The drawing under review shows one solid part. Ordinate dimensions are in mm from its lowest x, y, z. A direction names the side the tool comes from. Give positions to 0.01 mm unless a question says otherwise; leave off trailing zeros. Write each loop counter-clockwise with the first axis right and the second up, starting at its lowest first coordinate (ties: lowest second). Pieces come first, ordered by that corner, then holes. Notation, with made-up numbers: M -12.5,28.5 L 7.5,28.5 A9 ccw 7.5,45.5 Z; hole C -36,-12.75 d9. An arc over 180 degrees is marked long. Answer as a JSON object with one key per item and string values. Group by question number.
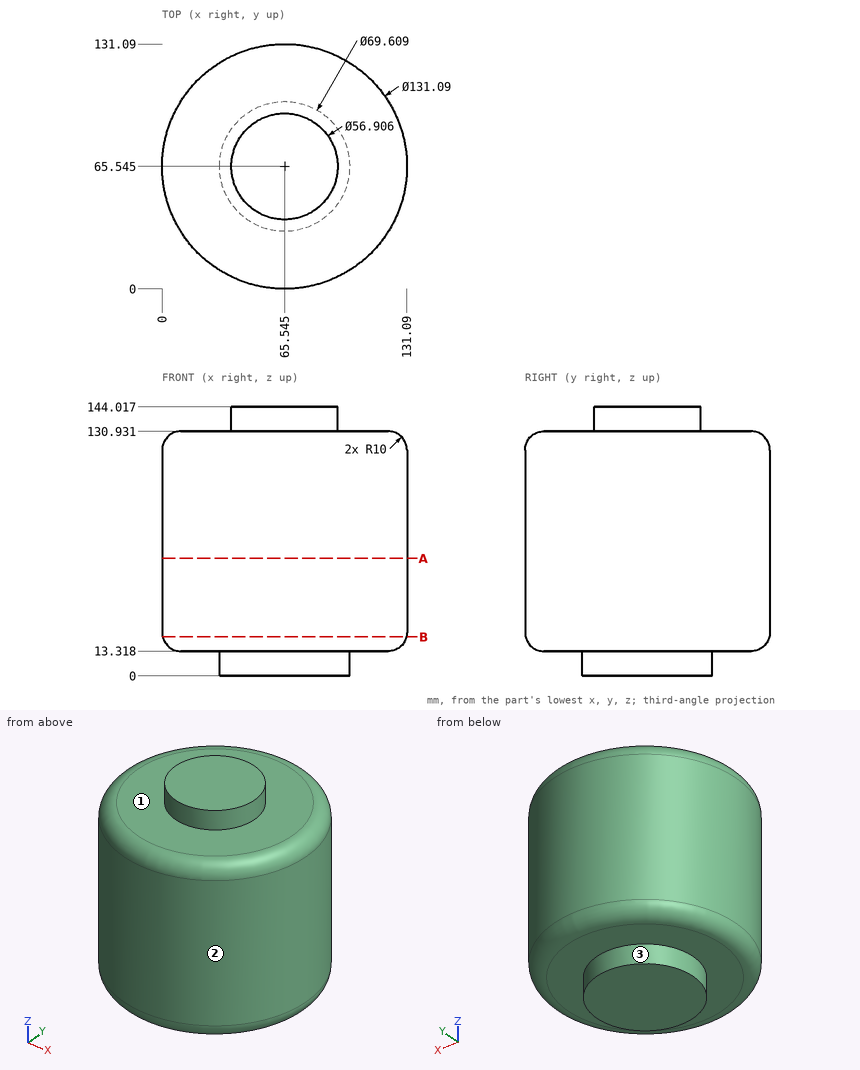
Item 1: Consider section B-B (z = 21). Give the boundary of the cut face in (x, y) (1 decimal).
Item 2: Insertion check: P1, Ø8, axis at x = 17, z = 69, coming from the +Y side; P2, Ø1.5, axis at x = 112, z = 125, coming from the +Y side (1 decimal); P3, Ø4, axis at x = 66, z = 120.5, coming from the -Y side. Each pin has a flat end and moves straight along its axis. Give the tip position at first contact, or say it passes through.
Item 3: To check wall thickness, follow probe 1 along Z at (x, y) = (47, 34.5); probe 2 along Y at (x, z) = (66, 110); probe 3 along Y at (x, z) = (11, 114.5). State the ranges of each line that lie inside material, in increasing order.
Item 4: Machinability: for the marked faces 1, 2 and 3, which of the approach directions +Z, -Z, +X, -X, +Y, -Y give a long, thin tool a straight path to every point of the face, cutting with its end or side? Answer none if there is none.
Item 5: Consider section A-A (z = 63). Give the boundary of the cut face in (x, y) (1 decimal).
Result set:
{
 "1": {"outline": "C 65.5,65.5 d130.5"},
 "2": {"P1": "stops at y = 113.63", "P2": "stops at y = 111.4", "P3": "stops at y = 0"},
 "3": {"probe 1": "z = 13.32 to 130.93", "probe 2": "y = 0 to 131.09", "probe 3": "y = 29.2 to 101.89"},
 "4": {"face 1": "+Z", "face 2": "+Z, -Z", "face 3": "-Z"},
 "5": {"outline": "C 65.5,65.5 d131.1"}
}
